Check sheet for the modelled part. Datum: model origin and axes. Units: mm. A direction names the side the tool comes from. Give positions to 0.01 mm unless a question says otherwise; leave off trailing zeros. Order: outer loops, then holes, each group sorted by start corner. A loop starts at its lowest first (then second) coordinate and runs counter-clockwise, first axis right, second up. Notation, with made-up numbers: (43.25, -4) -> (84.25, -4) arc R25 cw to (84.25, 16) -> close; hole circle Ø11 at (87, -19.5). An arc over 180 degrees is marked (long way). Answer in a Markdown table with one row per item. Add a question column.
(1) Go/stop test with flat-tipped pins: pin 1 (4 mm diameter, centred on x = 3.5, y = -5, fed in from +Z); pin 2 (6 mm diameter, centred on y = -0.5, z = 6, fed in from -X) (3 decimals); pin 3 (1.5 mm diameter, centred on y = -3.5, z = 8, fed in from +X). Record where each tip stops, or that it passes through.
(2) Cross-section at B-B (x = 2.5). Record the cut outline in (y, z) (3 decimals), then the cut area to 3 significant figures.
(3) Cross-section at D-D (z = 6.75). Record the cut outline in (x, y) (3 decimals), then the cut area to 3 significant figures.
(4) Set-up check for faces 1 (the face through (-2.975, 0, 6)), 2 (the face through (-4, 0, 0)), 3 (the face through (-4.808, 6.778, -6.36)): record each of +Z, -Z, +X, -X, +Y, -Y from which the full face is reachable in a straight line by a thin tool's end or side.
(5) Thickness scan on L1, parallel to Z at x = 4.25, y = -2.75; L2, parallel to Y at x = 1.5, z = 3; L3, parallel to Y at x = -0.5, z = 11. Record the ranges inside material, lowest first. Write a range as [from, to].
(6) Cross-section at A-A (z = -5.5). Record the cut outline in (x, y) (3 decimals).
(7) Cross-section at C-C (y = 4.5). Record the cut outline in (x, z) (3 decimals).
```python
from build123d import *

# Parameters (mm, degrees)
F1_DEPTH = 12.6
F2_DEPTH = 12.6
F4_DEPTH = 12.9


with BuildPart() as f1:
    # F0 (on Top) → F1 (new body)
    with BuildSketch(Plane.XY):
        with BuildLine():
            Line((-2.975, 0), (3.975, 0))
            ThreePointArc((3.975, 0), (1.409787, 3.716601), (-2.975, 2.636285))
            Line((-2.975, 2.636285), (-2.975, 0))
        make_face()
        with BuildLine():
            ThreePointArc((-2.975, -2.636285), (1.409787, -3.716601), (3.975, 0))
            Line((3.975, 0), (-2.975, 0))
            Line((-2.975, 0), (-2.975, -2.636285))
        make_face()
        with BuildLine():
            Line((-2.975, 0), (-2.975, 2.636285))
            ThreePointArc((-2.975, 2.636285), (-3.975, 0), (-2.975, -2.636285))
            Line((-2.975, -2.636285), (-2.975, 0))
        make_face()
    extrude(amount=F1_DEPTH)

    # F0 (on Top) → F2 (cut)
    with BuildSketch(Plane.XY):
        with BuildLine():
            Line((-2.975, 0), (-2.975, 2.636285))
            ThreePointArc((-2.975, 2.636285), (-3.975, 0), (-2.975, -2.636285))
            Line((-2.975, -2.636285), (-2.975, 0))
        make_face()
    extrude(amount=F2_DEPTH, mode=Mode.SUBTRACT)

    # F3 (on face) → F4 (join)
    with BuildSketch(Plane.XY):
        Polygon((5.525, 6.060786), (4.110786, 7.475), (-4.110786, 7.475), (-5.525, 6.060786), (-5.525, -6.060786), (-4.110786, -7.475), (4.110786, -7.475), (5.525, -6.060786), align=None)
    extrude(amount=-F4_DEPTH)


solid = f1.part
```
Answer below:
| question | item | result |
|---|---|---|
| 1 | pin 1 | stops at z = 0 |
| 1 | pin 2 | stops at x = -2.975 |
| 1 | pin 3 | stops at x = 2.87 |
| 2 | outline | (-7.475, -12.9) -> (7.475, -12.9) -> (7.475, 0) -> (3.09, 0) -> (3.09, 12.6) -> (-3.09, 12.6) -> (-3.09, 0) -> (-7.475, 0) -> close |
| 2 | area | 271 mm² |
| 3 | outline | (-2.975, -2.636) arc R3.975 ccw (long way) to (-2.975, 2.636) -> close |
| 3 | area | 46.0 mm² |
| 4 | face 1 | +Z, -X, +Y, -Y |
| 4 | face 2 | +Z |
| 4 | face 3 | +Z, -Z, -X, +Y |
| 5 | L1 | z = [-12.9, 0] |
| 5 | L2 | y = [-3.68, 3.68] |
| 5 | L3 | y = [-3.94, 3.94] |
| 6 | outline | (-5.525, -6.061) -> (-4.111, -7.475) -> (4.111, -7.475) -> (5.525, -6.061) -> (5.525, 6.061) -> (4.111, 7.475) -> (-4.111, 7.475) -> (-5.525, 6.061) -> close |
| 7 | outline | (-5.525, -12.9) -> (5.525, -12.9) -> (5.525, 0) -> (-5.525, 0) -> close |
